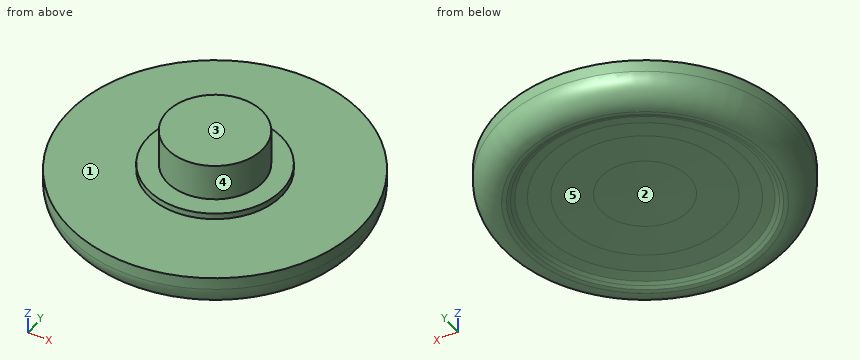
```python
from build123d import *

# Parameters (mm, degrees)
F0_R     = 12
F1_DEPTH = 2
F2_R     = 12
F2_R_2   = 10
F3_DEPTH = 1
F4_R     = 1.99999
F5_R     = 5.5
F6_DEPTH = 0.5
F7_R     = 3.925
F8_DEPTH = 3


# Not quite as in the source:
# - a fillet or chamfer is up to 0.001 mm smaller than in the source, because OpenCascade refuses the exact size


with BuildPart() as f1:
    # F0 (on Top) → F1 (new body)
    with BuildSketch(Plane.XY):
        Circle(F0_R)
    extrude(amount=F1_DEPTH)

    # F2 (on face) → F3 (join)
    with BuildSketch(Plane(origin=(0, 0, 0), x_dir=(1, 0, 0), z_dir=(0, 0, -1))):
        Circle(F2_R)
        Circle(F2_R_2, mode=Mode.SUBTRACT)
    extrude(amount=F3_DEPTH)

    # F4 (radius 2 in the source; OpenCascade refuses exactly that, so slightly less here)
    f4_edges = [f1.edges().sort_by_distance(p)[0] for p in [
        (-12, 0, -1),
    ]]
    fillet(f4_edges, radius=F4_R)

    # F5 (on face) → F6 (join)
    with BuildSketch(Plane.XY.offset(2)):
        Circle(F5_R)
    extrude(amount=F6_DEPTH)

    # F7 (on face) → F8 (join)
    with BuildSketch(Plane.XY.offset(2.5)):
        Circle(F7_R)
    extrude(amount=F8_DEPTH)

    # F9 (on Front) → F10 (revolve)
    with BuildSketch(Plane.XZ):
        Polygon((-10.0021678954, 0), (-10.0021678954, -1.0005384684), (-9.6580199897, -0.9450307698), (-9.385343641, -0.8195927949), (-9.0745007619, -0.6752727786), (-8.19747895, -0.5198512226), (-6.5711033531, -0.3644296667), (-3.5958907101, -0.2090081107), (0, -0.0646880944), (0, 0), align=None)
    revolve(axis=Axis((0, 0, -0.0323440472), (0, 0, 1)))


solid = f1.part
```
The model under review builds one solid part; all positions refer to its coordinate system, in mm. Face numbers are marked on the shaded views. A direction names the side the tool comes from. Round coordinates to 2 decimals unless told otherwise and drop trailing zeros. Order: outer loops, then holes, each group sorted by start corner. A loop starts at its lowest first (then second) coordinate and runs counter-clockwise, first axis right, second up. Notation, with made-up numbers: (3, -13) -> (28, -13) arc R10 ccw to (28, 0) -> close; hole circle Ø3 at (67.5, 33). An arc over 180 degrees is marked (long way). Use a Markdown table: item, result.
Q1. Mouldability with a two-part tool opening along X and no side actions: class the marked faces 3, 4 and 5 as +X half, -X half, draft (parallel to the pull), parting line (faces both ways), or undercut.
Values:
| item | result |
|---|---|
| face 3 | draft |
| face 4 | parting line |
| face 5 | undercut |
Q2. Clearance check with a flat-ended pin moving along its axis: P1, Ø3, axis at x = -3.5, y = -2, coming from the -Z side. State where the tip first meets the part, or that it passes through.
Values:
| item | result |
|---|---|
| P1 | stops at z = -0.31 |
Q3. Tool access review of the marked faces 1 and 2: name each direction out of +Z, -Z, +X, -X, +Y, -Y from which nothing blocks a thin tool from reaching the whole face with its end or side.
Values:
| item | result |
|---|---|
| face 1 | +Z |
| face 2 | -Z |
Q4. We need section A-A on z = 4. Write out the cut boundary in (x, y) (3 decimals), then the cut area to 3 significant figures.
Values:
| item | result |
|---|---|
| outline | circle Ø7.85 at (0, 0) |
| area | 48.4 mm^2 |
Q5. For line 1 (Z direction, x = -3.75, y = 9.25); line 2 (X direction, y = -2, z = 0.75); line 3 (X direction, y = -1.75, z = 2.25), list the stretches that pass through material, from the lowest coordinate up.
Values:
| item | result |
|---|---|
| line 1 | z = -1 to 2 |
| line 2 | x = -11.82 to 11.82 |
| line 3 | x = -5.21 to 5.21 |
